Solid Edge part; units mm, degrees
sketch "Sketch1" plane through (0, 0, 0) normal (0, -1, 0) x (1, 0, 0)
  line L0 (-6, 8) -> (6, 8)
  line L1 (6, 8) -> (6, 0)
  line L2 (6, 0) -> (-6, 0)
  line L3 (-6, 0) -> (-6, 8)
  dimension "D1" = 6
  dimension "D2" = 6
extrude "Protrusion1" add sketch "Sketch1" along normal mid plane 420
sketch "Sketch2" plane through (0, 0, 8) normal (0, 0, 1) x (0, 1, 0)
  circle A0 centre (200, 0) radius 1.75
extrude "Cutout1" cut sketch "Sketch2" against normal through all
sketch "Sketch3" plane through (0, 0, 8) normal (0, 0, 1) x (0, 1, 0)
  circle A0 centre (200, 0) radius 3
extrude "ExtrudedCutout_2" cut sketch "Sketch3" against normal blind 4.5
pattern_linear "Pattern1" count 17 spacing 25 along (0, -1, 0) of "Cutout1", "ExtrudedCutout_2"
properties material "Stainless Steel, 410"
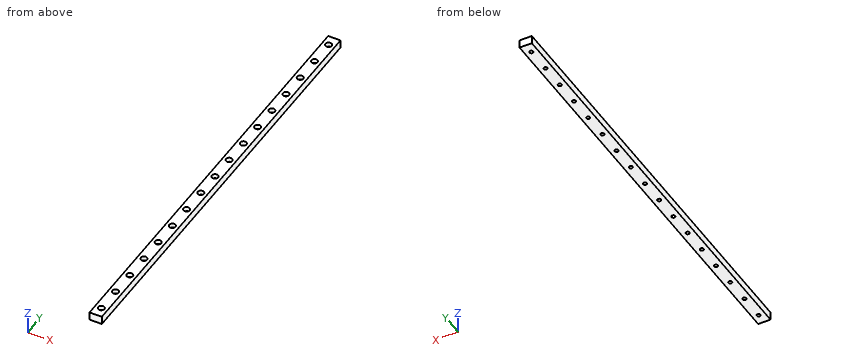
Here's how the part is built. I have some questions about the finished solid (model axes, mm). Coordinates: 2 decimals unless noted, no trailing zeros. Return JSON: item names as keys, results as strings. Group by question number.
Item 1: I need wall thicknesses on line 1 (X direction, y = -200, z = 2.65); line 2 (X direction, y = -175, z = 6.25); line 3 (Z direction, x = -2.5, y = -173.5). Which ranges of each line are inside material? Lowest first, please. Write a range as from..to.
Item 2: If we section it at A-A on z = 1.5: State how many separate pieces and enclosed holes the cut face has, and give its area (3 significant figures).
Item 3: Will these pins go through, and if not, where does the flat tip stop? P1, Ø4, axis at x = -4.5, y = 96.5, coming from the -Z side; P2, Ø4, axis at x = 0, y = 125, coming from the +Z side.
Calculated:
{
 "1": {"line 1": "x = -6..-1.75, 1.75..6", "line 2": "x = -6..-3, 3..6", "line 3": "z = 0..3.5"},
 "2": {"separate pieces": "1", "enclosed holes": "17", "area": "4,880 mm^2"},
 "3": {"P1": "stops at z = 0", "P2": "stops at z = 3.5"}
}
